Design review of the part built by this model. Coordinates are the model's own, in mm. Give positions to 0.01 mm unless a question says otherwise; leave off trailing zeros. Order: outer loops, then holes, each group sorted by start corner. A loop starts at its lowest first (then second) coordinate and runs counter-clockwise, first axis right, second up. Notation, with made-up numbers: (13.25, 60.25) -> (60.25, 60.25) arc R29 cw to (60.25, 90.25) -> close; hole circle Ø7 at (39.25, -9.5). An arc over 180 degrees is marked (long way). Return JSON: item names as keys, results as strings.
```python
from build123d import *

# Parameters (mm, degrees)
F1_W     = 40
F1_H     = 19
F3_DEPTH = 1275
F2_W     = 80
F2_H     = 100
F4_DEPTH = 25
F6_DEPTH = 40


with BuildPart() as f3:
    # F1 (on Right) → F3 (new body, symmetric)
    with BuildSketch(Plane.YZ):
        Polygon((20, 33), (20, 63), (17, 66), (12, 66), (12, 80), (4, 80), (4, 66), (-4, 66), (-4, 80), (-12, 80), (-12, 66), (-17, 66), (-20, 63), (-20, 33), align=None)
        with Locations((0, 23.5)):
            Rectangle(F1_W, F1_H)
    extrude(amount=F3_DEPTH, both=True)

    # F2 (on Front) → F4 (cut, symmetric)
    with BuildSketch(Plane.XZ):
        with Locations((-1275, 83)):
            Rectangle(F2_W, F2_H)
        with Locations((-1275, -83)):
            Rectangle(F2_W, F2_H)
        with Locations((1275, 83)):
            Rectangle(F2_W, F2_H)
        with Locations((1275, -83)):
            Rectangle(F2_W, F2_H)
    extrude(amount=F4_DEPTH, both=True, mode=Mode.SUBTRACT)

    # F5 (on face) → F6 (cut, through all)
    with BuildSketch(Plane.XZ.offset(20)):
        Polygon((-1235, 33), (-1275, 33), (-1275, 14), (1275, 14), (1275, 33), (1235, 33), align=None)
    extrude(amount=-F6_DEPTH, mode=Mode.SUBTRACT)


solid = f3.part
```
Item 1: Wall thickness on L1, parallel to Y at x = 696, z = 73.5; L2, parallel to Z at x = -1128, y = -14.5; L3, parallel to Y at x = 417.5, z = 65: over which ranges is each line inside the solid? List them lowest first. Write a range as [from, to].
Result set:
{"L1": "y = [-12, -4], [4, 12]", "L2": "z = [33, 66]", "L3": "y = [-18, 18]"}
Item 2: For pin 1 (11 mm diameter, centred on x = -515, z = 76, fed in from +Y); pin 2 (11 mm diameter, centred on x = -546.5, z = 75.5, fed in from -Y); pin 3 (2 mm diameter, centred on x = -254, y = 14.5, fed in from +Z), all flat-tipped, find the tip position at first contact; note any pin that passes through.
Result set:
{"pin 1": "stops at y = 12", "pin 2": "stops at y = -12", "pin 3": "stops at z = 66"}
Item 3: Add section A-A (x = 79). Give the boundary of the cut face in (y, z).
Result set:
{"outline": "(-20, 33) -> (20, 33) -> (20, 63) -> (17, 66) -> (12, 66) -> (12, 80) -> (4, 80) -> (4, 66) -> (-4, 66) -> (-4, 80) -> (-12, 80) -> (-12, 66) -> (-17, 66) -> (-20, 63) -> close"}
